```python
from build123d import *

# Parameters (mm, degrees)
BOSS_EXTRUDE1_DEPTH = 7
SKETCH2_R           = 7
CUT_EXTRUDE1_DEPTH  = 5
SKETCH3_R           = 1.5
CUT_EXTRUDE2_DEPTH  = 5
FILLET1_R           = 0.5


with BuildPart() as part:
    # Sketch1 → Boss-Extrude1 (new body)
    with BuildSketch(Plane.XY):
        with BuildLine():
            ThreePointArc((0, 11), (-7.778174593, 7.778174593), (-11, 0))
            ThreePointArc((-11, 0), (-7.778174593, -7.778174593), (0, -11))
            Line((0, -11), (0, -4))
            ThreePointArc((0, -4), (-4, 0), (0, 4))
            Line((0, 4), (0, 11))
        make_face()
        with BuildLine():
            ThreePointArc((11, 0), (7.778174593, 7.778174593), (0, 11))
            Line((0, 11), (0, 4))
            ThreePointArc((0, 4), (2.828427125, 2.828427125), (4, 0))
            ThreePointArc((4, 0), (2.828427125, -2.828427125), (0, -4))
            Line((0, -4), (0, -11))
            ThreePointArc((0, -11), (7.778174593, -7.778174593), (11, 0))
        make_face()
        with BuildLine():
            ThreePointArc((0, -11), (-7.778174593, -7.778174593), (-11, 0))
            Line((-11, 0), (-11, -8))
            Line((-11, -8), (-20, -8))
            Line((-20, -8), (-20, -13))
            Line((-20, -13), (0, -13))
            Line((0, -13), (0, -11))
        make_face()
        with BuildLine():
            ThreePointArc((11, 0), (7.778174593, -7.778174593), (0, -11))
            Line((0, -11), (0, -13))
            Line((0, -13), (20, -13))
            Line((20, -13), (20, -8))
            Line((20, -8), (11, -8))
            Line((11, -8), (11, 0))
        make_face()
    extrude(amount=BOSS_EXTRUDE1_DEPTH)

    # Sketch2 → Cut-Extrude1 (cut)
    with BuildSketch(Plane(origin=(0, 0, 0), x_dir=(-1, 0, 0), z_dir=(0, 0, -1))):
        Circle(SKETCH2_R)
    extrude(amount=-CUT_EXTRUDE1_DEPTH, mode=Mode.SUBTRACT)

    # Sketch3 → Cut-Extrude2 (cut)
    with BuildSketch(Plane(origin=(0, -8, 0), x_dir=(1, 0, 0), z_dir=(0, 1, 0))):
        with Locations(Location((-15.5, -3.5, 0), (0, 0, 270))):
            Circle(SKETCH3_R)
        with Locations(Location((15.5, -3.5, 0), (0, 0, 90))):
            Circle(SKETCH3_R)
    extrude(amount=-CUT_EXTRUDE2_DEPTH, mode=Mode.SUBTRACT)

    # Fillet1
    fillet1_edges = [part.edges().sort_by_distance(p)[0] for p in [
        (20, -10.5, 7),
        (-20, -10.5, 0),
        (20, -10.5, 0),
        (-20, -10.5, 7),
    ]]
    fillet(fillet1_edges, radius=FILLET1_R)


solid = part.part
```
The model under review builds one solid part; all positions refer to its coordinate system, in mm. A direction names the side the tool comes from. Round coordinates to 2 decimals unless told otherwise and drop trailing zeros. Loops run counter-clockwise (first coordinate to the right, second up) from the corner with the lowest first, then second, coordinate; pieces in that order, holes last. Notation, with made-up numbers: M 56,25 L 114,25 A8 ccw 114,39 Z; hole C -6.5,37.25 d11. An arc over 180 degrees is marked long. Write item = value, one per line.
Item 1: Take a section at A-A on z = 3.5. Write out the cut boundary in (x, y).
Return value:
outline = M -20,-13 L -17,-13 L -17,-8 L -20,-8 Z; M -14,-13 L 14,-13 L 14,-8 L 11,-8 L 11,0 A11 ccw -11,0 L -11,-8 L -14,-8 Z; M 17,-13 L 20,-13 L 20,-8 L 17,-8 Z; hole C 0,0 d14
Item 2: Take a section at D-D on y = -11.25. Write out the cut boundary in (x, z), then the cut area to 3 significant figures.
Return value:
outline = M -20,0.5 A0.5 ccw -19.5,0 L 19.5,0 A0.5 ccw 20,0.5 L 20,6.5 A0.5 ccw 19.5,7 L -19.5,7 A0.5 ccw -20,6.5 Z; hole C -15.5,3.5 d3; hole C 15.5,3.5 d3
area = 266 mm2
Item 3: Machinability: for faces 1 (the flat face through (0, -6, 7)), 2 (the flat face through (-16.4, -8, 5)), 3 (the cylindrical face through (-6.466, -2.681, 2.465)), 4 (the flat face through (17, -8, 5)), which of the approach directions +Z, -Z, +X, -X, +Y, -Y give a long, thin tool a straight path to every point of the face, cutting with its end or side? Answer none if there is none.
Return value:
face_1 = +Z, +X, -X, +Y, -Y
face_2 = +Z, -Z, -X, +Y
face_3 = -Z
face_4 = +Z, -Z, +X, +Y
Item 4: Take a section at B-B on x = -15.5. Write out the cut boundary in (y, z), then the cut area to 3 significant figures.
Return value:
outline = M -13,0 L -8,0 L -8,2 L -13,2 Z; M -13,5 L -8,5 L -8,7 L -13,7 Z
area = 20.0 mm2
Item 5: Insertion check: P1, Ø2.5, axis at x = 15.5, z = 3.5, coming from the -Y side; P2, Ø3, axis at y = -0.5, z = 5.5, coming from the +X side; P3, Ø1.5, axis at y = -4, z = 1.5, coming from the -X side. Each pin has a flat end and moves straight along its axis. Give the tip position at first contact, or say it passes through.
Return value:
P1 = through
P2 = 11
P3 = -11
Item 6: Take a section at C-C on z = 1. Write out the cut boundary in (x, y), then the cut area to 3 significant figures.
Return value:
outline = M -20,-13 L 20,-13 L 20,-8 L 11,-8 L 11,0 A11 ccw -11,0 L -11,-8 L -20,-8 Z; hole C 0,0 d14
area = 412 mm2
Item 7: For line 1 (X direction, y = -11.4, z = 3.5); line 2 (Y direction, x = 0, z = 2.75); line 3 (Z direction, x = 15.5, y = -9.85), list the stretches that pass through material, from the lowest coordinate up. Write a range as [from, to].
Return value:
line_1 = [-20, -17], [-14, 14], [17, 20]
line_2 = [-13, -7], [7, 11]
line_3 = [0, 2], [5, 7]
Item 8: The part is to be moulded in two halves that separate along X. For faces 5 (the flat face through (11, -4, 3)), 6 (the cylindrical face through (15.05, -10.46, 2.07)), 7 (the flat face through (0, -13, 3)), say which applies: released by +X, released by -X, zero draft, split by the parting line, or undercut.
Return value:
face_5 = released by +X
face_6 = undercut
face_7 = zero draft
